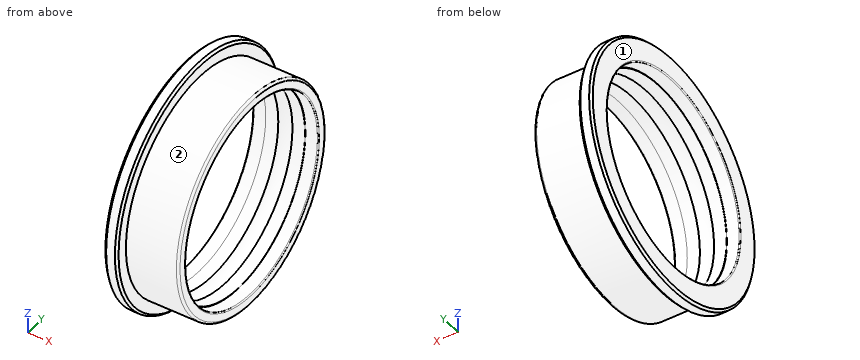
Autodesk Inventor part; units mm, degrees
ref_plane "1_XY" through (1.5, 0, 0) normal (1, 0, 0) x (0, 0, -1)
ref_plane "1_YZ" through (1.5, 0, 0) normal (0, 0, -1) x (0, 1, 0)
ref_plane "1_ZX" through (1.5, 0, 0) normal (0, 1, 0) x (1, 0, 0)
sketch "Sketch_3" plane through (0, 0, 0) normal (0, 0, 1) x (1, 0, 0)
  line L0 (2.9, 0) -> (0, 0)
  line L1 (0, 5.5) -> (0, 4.57)
  arc A0 (0, 4.57) -> (0.05, 4.52) centre (0.05, 4.57) ccw
  line L2 (0.05, 4.52) -> (0.605, 4.52)
  line L3 (0.605, 4.52) -> (0.605, 4.5001)
  line L4 (0.605, 4.5001) -> (1.177, 4.5001)
  arc A1 (1.823, 4.5001) -> (1.177, 4.5001) centre (1.5, 4) ccw
  line L5 (1.823, 4.5001) -> (2.4, 4.5001)
  line L6 (2.4, 4.5001) -> (2.4, 4.52)
  line L7 (2.4, 4.52) -> (2.95, 4.52)
  arc A2 (2.95, 4.52) -> (3, 4.57) centre (2.95, 4.57) ccw
  line L8 (3, 4.57) -> (3, 4.9)
  arc A3 (3, 4.9) -> (2.9, 5) centre (2.9, 4.9) ccw
  line L9 (2.9, 5) -> (0.6, 5)
  line L10 (0.6, 5) -> (0.6, 5.5)
  line L11 (0.6, 5.5) -> (0.5, 5.6)
  line L12 (0.5, 5.6) -> (0.1, 5.6)
  line L13 (0.1, 5.6) -> (0, 5.5)
revolve "Revolution1" add sketch "Sketch_3" angle 360 about axis through (2.9, 0, 0) along (1, 0, 0)
ref_plane "1_XY" through (1.5, 0, 0) normal (1, 0, 0) x (0, 0, -1)
ref_plane "1_YZ" through (1.5, 0, 0) normal (0, 0, -1) x (0, 1, 0)
ref_plane "1_ZX" through (1.5, 0, 0) normal (0, 1, 0) x (1, 0, 0)
properties part number "LF-1060ZZ_or" material "鋼、炭素鋼"
Source: CAD feature listing. Evaluate the final solid. Frame: model axes, mm. Face numbers are marked on the shaded views. A direction names the side the tool comes from. Give positions to 0.01 mm unless a question says otherwise; leave off trailing zeros. Order: outer loops, then holes, each group sorted by start corner. A loop starts at its lowest first (then second) coordinate and runs counter-clockwise, first axis right, second up. Notation, with made-up numbers: (-34, 9) -> (-4, 9) arc R26 cw to (-4, 40) -> close; hole circle Ø4 at (89, 14.25). An arc over 180 degrees is marked (long way). Use a Markdown table: item, result.
Q1. Access query for the marked faces 1 and 2. Directions: +Z, -Z, +X, -X, +Y, -Y. A direction counts if a zero-diameter tool reaches every point of the face in a straight line with its end or side. Return the directions, or none.
A:
| item | result |
|---|---|
| face 1 | +Z, -Z, -X, +Y, -Y |
| face 2 | +X |
Q2. First-contact query: P1, Ø1.5, axis at x = 0.5, y = 3.5, coming from the +Z side; P2, Ø1.5, axis at x = 1, z = -4.5, coming from the +Y side. Flat tips, straight axial feed; report the tip coordinate or a pass-through.
A:
| item | result |
|---|---|
| P1 | z = 4.88 |
| P2 | y = 3.98 |
Q3. Material intervals for line 1 (Z direction, x = 2.6, y = 0); line 2 (X direction, y = -3, z = 4.5); line 3 (Z direction, x = 0.3, y = 0), sorted ascending. Write a range as [from, to].
A:
| item | result |
|---|---|
| line 1 | [-5, -4.52], [4.52, 5] |
| line 2 | [0, 0.6] |
| line 3 | [-5.6, -4.52], [4.52, 5.6] |
Q4. Section C-C (x = 1). Return the cut outline in (y, z), and give its area (3 significant figures).
A:
| item | result |
|---|---|
| outline | circle Ø10 at (0, 0); hole circle Ø9 at (0, 0) |
| area | 14.9 mm^2 |
